```python
from build123d import *

# Parameters (mm, degrees)
SKETCH1_R           = 16
SKETCH1_R_2         = 9.5
BOSS_EXTRUDE1_DEPTH = 6
SKETCH1_3_R         = 25
SKETCH1_3_R_2       = 2.5
SKETCH1_3_R_3       = 16
BOSS_EXTRUDE2_DEPTH = 4


with BuildPart() as part:
    # Sketch1 → Boss-Extrude1 (new body)
    with BuildSketch(Plane(origin=(0, 0, 0), x_dir=(0, 1, 0), z_dir=(0, 0, 1))):
        with Locations(Location((0, 0, 0), (0, 0, 270))):
            Circle(SKETCH1_R)
        with Locations(Location((-5, 0, 0), (0, 0, 270))):
            Circle(SKETCH1_R_2, mode=Mode.SUBTRACT)
    extrude(amount=BOSS_EXTRUDE1_DEPTH)

    # Sketch1_3 → Boss-Extrude2 (add)
    with BuildSketch(Plane(origin=(0, 0, 0), x_dir=(0, 1, 0), z_dir=(0, 0, 1))):
        with Locations(Location((0, 0, 0), (0, 0, 270))):
            Circle(SKETCH1_3_R)
        with Locations(Location((-7.845010363, 18.939530416, 0), (0, 0, 270))):
            Circle(SKETCH1_3_R_2, mode=Mode.SUBTRACT)
        with Locations(Location((-14.495689014, 14.495689014, 0), (0, 0, 270))):
            Circle(SKETCH1_3_R_2, mode=Mode.SUBTRACT)
        with Locations(Location((-18.939530416, 7.845010363, 0), (0, 0, 270))):
            Circle(SKETCH1_3_R_2, mode=Mode.SUBTRACT)
        with Locations(Location((-20.5, 0, 0), (0, 0, 270))):
            Circle(SKETCH1_3_R_2, mode=Mode.SUBTRACT)
        with Locations(Location((-18.939530416, -7.845010363, 0), (0, 0, 270))):
            Circle(SKETCH1_3_R_2, mode=Mode.SUBTRACT)
        with Locations(Location((-14.495689014, -14.495689014, 0), (0, 0, 270))):
            Circle(SKETCH1_3_R_2, mode=Mode.SUBTRACT)
        with Locations(Location((-7.845010363, -18.939530416, 0), (0, 0, 270))):
            Circle(SKETCH1_3_R_2, mode=Mode.SUBTRACT)
        with Locations(Location((0, -20.5, 0), (0, 0, 270))):
            Circle(SKETCH1_3_R_2, mode=Mode.SUBTRACT)
        with Locations(Location((7.845010363, -18.939530416, 0), (0, 0, 270))):
            Circle(SKETCH1_3_R_2, mode=Mode.SUBTRACT)
        with Locations(Location((14.495689014, -14.495689014, 0), (0, 0, 270))):
            Circle(SKETCH1_3_R_2, mode=Mode.SUBTRACT)
        with Locations(Location((18.939530416, -7.845010363, 0), (0, 0, 270))):
            Circle(SKETCH1_3_R_2, mode=Mode.SUBTRACT)
        with Locations(Location((20.5, 0, 0), (0, 0, 270))):
            Circle(SKETCH1_3_R_2, mode=Mode.SUBTRACT)
        with Locations(Location((18.939530416, 7.845010363, 0), (0, 0, 270))):
            Circle(SKETCH1_3_R_2, mode=Mode.SUBTRACT)
        with Locations(Location((14.495689014, 14.495689014, 0), (0, 0, 270))):
            Circle(SKETCH1_3_R_2, mode=Mode.SUBTRACT)
        with Locations(Location((7.845010363, 18.939530416, 0), (0, 0, 270))):
            Circle(SKETCH1_3_R_2, mode=Mode.SUBTRACT)
        with Locations(Location((0, 20.5, 0), (0, 0, 270))):
            Circle(SKETCH1_3_R_2, mode=Mode.SUBTRACT)
        with Locations(Location((0, 0, 0), (0, 0, 270))):
            Circle(SKETCH1_3_R_3, mode=Mode.SUBTRACT)
    extrude(amount=BOSS_EXTRUDE2_DEPTH)


solid = part.part
```
Geometry: final body of the model. Coordinates: model frame, mm. A direction names the side the tool comes from. Give positions to 0.01 mm unless a question says otherwise; leave off trailing zeros. Order: outer loops, then holes, each group sorted by start corner. A loop starts at its lowest first (then second) coordinate and runs counter-clockwise, first axis right, second up. Notation, with made-up numbers: (11, -22) -> (49, -22) arc R27 ccw to (49, -6) -> close; hole circle Ø9 at (-33, 11.5). An arc over 180 degrees is marked (long way). Write each question's results on one line, items separated by ' | '. Start each with the question number.
1) Section A-A (x = 0). Return loops of the section in (y, z).
2) Set-up query: faces 1 (the flat face through (-0.4, -16.3, 4)), 2 (the cylindrical face through (12.5, -16, 2)). Return all of +Z, -Z, +X, -X, +Y, -Y with unobstructed straight access to the full face (end or side cutting, diameter ignored); none if empty.
3) Section B-B (x = -13.5). Return loops of the section in (y, z).
4) Draft query along X for faces 3 (the cylindrical face through (-3.47, -15.62, 4.99)), 4 (the cylindrical face through (7.52, -16.46, 1.97)), 5 (the flat face through (-4, 4, 6)). Return one class per face: pulls with the +X half, pulls with the -X half, needs draft (parallel to the pull), parting line crosses it, or undercut.
5) Section D-D (z = 5.3). Return loops of the section in (x, y), then the cut area to 3 significant figures.
6) Line query: line 1 (Y direction, x = 7, z = 0.6); line 2 (X direction, y = -15.5, z = 2.45); line 3 (X direction, y = 0.5, z = 0.4) (3 decimals). Output: solid intervals per line, ascending. Write a range as from..to.
7) First-contact query: pin 1 (5 mm diameter, centred on x = 9.5, y = 8, fed in from -Z); pin 2 (6 mm diameter, centred on x = 14.5, y = -14.5, fed in from +Z); pin 3 (1.5 mm diameter, centred on y = -13.5, z = 1, fed in from +X); pin 4 (1.5 mm diameter, centred on y = 11, z = 4.5, fed in from +X). Flat tips, straight axial feed; report the tip coordinate or a pass-through.
8) Section C-C (y = 20.5). Return loops of the section in (x, z).
Calculated:
1) outline: (-25, 0) -> (-23, 0) -> (-23, 4) -> (-25, 4) -> close; (-18, 0) -> (-14.5, 0) -> (-14.5, 6) -> (-16, 6) -> (-16, 4) -> (-18, 4) -> close; (4.5, 0) -> (18, 0) -> (18, 4) -> (16, 4) -> (16, 6) -> (4.5, 6) -> close; (23, 0) -> (25, 0) -> (25, 4) -> (23, 4) -> close
2) face 1: +Z | face 2: +Z, -Z
3) outline: (-21.04, 0) -> (-16.79, 0) -> (-16.79, 4) -> (-21.04, 4) -> close; (-12.2, 0) -> (12.2, 0) -> (12.2, 4) -> (8.59, 4) -> (8.59, 6) -> (-8.59, 6) -> (-8.59, 4) -> (-12.2, 4) -> close; (16.79, 0) -> (21.04, 0) -> (21.04, 4) -> (16.79, 4) -> close
4) face 3: parting line crosses it | face 4: undercut | face 5: needs draft
5) outline: circle Ø32 at (0, 0); hole circle Ø19 at (0, -5) | area: 521 mm2
6) line 1: -24..-21.29, -16.59..-11.42, 1.42..16.59, 21.29..24 | line 2: -19.62..-16.79, -12.21..12.21, 16.79..19.62 | line 3: -24.995..-22.949, -18.051..-7.746, 7.746..18.051, 22.949..24.995
7) pin 1: z = 0 | pin 2: z = 4 | pin 3: x = 21.5 | pin 4: x = 22.72
8) outline: (-14.31, 0) -> (-9.8, 0) -> (-9.8, 4) -> (-14.31, 4) -> close; (-5.89, 0) -> (-2.5, 0) -> (-2.5, 4) -> (-5.89, 4) -> close; (2.5, 0) -> (5.89, 0) -> (5.89, 4) -> (2.5, 4) -> close; (9.8, 0) -> (14.31, 0) -> (14.31, 4) -> (9.8, 4) -> close
